Can you work these out from the model? Positions are in its coordinate system, mm. A direction names the side the tool comes from. Coordinates: 2 decimals unless noted, no trailing zeros. Order: outer loops, then holes, each group sorted by start corner. A loop starts at its lowest first (then second) coordinate and runs counter-clockwise, first axis right, second up. Notation, with made-up numbers: M 9.5,66.25 L 19.5,66.25 A22 cw 19.5,93.25 Z; hole C 53,15.25 d11. An arc over 180 degrees is marked long. Answer as a JSON object with one key per item and string values.
from build123d import *

# Parameters (mm, degrees)
SKETCH_1_W          = 29.8
SKETCH_1_H          = 29.8
SKETCH_1_W_2        = 25
SKETCH_1_H_2        = 25
EXTRUDE_1_DEPTH     = 40
SKETCH_2_R          = 8
SKETCH_2_R_2        = 5
EXTRUDE_1_2_DEPTH   = 10
SKETCH_3_R          = 8
EXTRUDE_2_DEPTH     = 4
FILLET_1_R          = 10
CUT_EXTRUDE_1_REACH = 58.671
SKETCH_4_R          = 2.2
SKETCH_5_R          = 5
CUT_EXTRUDE_2_DEPTH = 10
CUT_EXTRUDE_3_REACH = 52.454
SKETCH_6_W          = 25
SKETCH_6_H          = 25
SKETCH_7_R          = 3.2
SKETCH_7_R_2        = 1.2
EXTRUDE_3_DEPTH     = 4
FILLET_2_R          = 10


with BuildPart() as part:
    # Эскиз1 → Extrude 1 (new body)
    with BuildSketch(Plane(origin=(0, 0, 0), x_dir=(0, 0, -1), z_dir=(1, 0, 0))):
        Rectangle(SKETCH_1_W, SKETCH_1_H)
        Rectangle(SKETCH_1_W_2, SKETCH_1_H_2, mode=Mode.SUBTRACT)
    extrude(amount=EXTRUDE_1_DEPTH)

    # Эскиз2 → Extrude 1 2 (add)
    with BuildSketch(Plane(origin=(0, 14.9, 0), x_dir=(1, 0, 0), z_dir=(0, 1, 0))):
        with Locations((20, -18.9)):
            Circle(SKETCH_2_R)
        with Locations((20, -18.9)):
            Circle(SKETCH_2_R_2, mode=Mode.SUBTRACT)
    extrude(amount=-EXTRUDE_1_2_DEPTH)

    # Эскиз3 → Бобышка-Вытянуть2 (add)
    with BuildSketch(Plane.XZ.offset(-4.9)):
        with Locations((20, 18.9)):
            Circle(SKETCH_3_R)
    extrude(amount=EXTRUDE_2_DEPTH)

    # Скругление1
    fillet_1_edges = [part.edges().sort_by_distance(p)[0] for p in [
        (13.07179677, 7.9, 14.9),
        (26.92820323, 7.9, 14.9),
        (20, 0.9, 14.9),
    ]]
    fillet(fillet_1_edges, radius=FILLET_1_R)

    # Эскиз4 → Вырез-Вытянуть1 (cut, up to next)
    with BuildSketch(Plane(origin=(0, 14.9, 0), x_dir=(1, 0, 0), z_dir=(0, 1, 0)), mode=Mode.PRIVATE) as cut_extrude_1_sk1:
        with Locations(Location((10, 0, 0), (0, 0, 270))):
            Circle(SKETCH_4_R)
    cut_extrude_1_tool1 = extrude(cut_extrude_1_sk1.sketch, amount=-CUT_EXTRUDE_1_REACH, mode=Mode.PRIVATE) & part.part
    # Эскиз4 → Вырез-Вытянуть1 (cut, up to next)
    with BuildSketch(Plane(origin=(0, 14.9, 0), x_dir=(1, 0, 0), z_dir=(0, 1, 0)), mode=Mode.PRIVATE) as cut_extrude_1_sk2:
        with Locations(Location((30, 0, 0), (0, 0, 270))):
            Circle(SKETCH_4_R)
    cut_extrude_1_tool2 = extrude(cut_extrude_1_sk2.sketch, amount=-CUT_EXTRUDE_1_REACH, mode=Mode.PRIVATE) & part.part
    add(cut_extrude_1_tool1.solids().sort_by_distance((10, 14.9, 0))[0], mode=Mode.SUBTRACT)
    add(cut_extrude_1_tool2.solids().sort_by_distance((30, 14.9, 0))[0], mode=Mode.SUBTRACT)

    # Эскиз5 → Вырез-Вытянуть2 (cut)
    with BuildSketch(Plane(origin=(0, 14.9, 0), x_dir=(1, 0, 0), z_dir=(0, 1, 0))):
        with Locations(Location((20, -18.9, 0), (0, 0, 270))):
            Circle(SKETCH_5_R)
    extrude(amount=-CUT_EXTRUDE_2_DEPTH, mode=Mode.SUBTRACT)

    # Эскиз6 → Вырез-Вытянуть3 (cut, up to next)
    with BuildSketch(Plane(origin=(40, 0, 0), x_dir=(0, 0, -1), z_dir=(1, 0, 0)), mode=Mode.PRIVATE) as cut_extrude_3_sk1:
        Rectangle(SKETCH_6_W, SKETCH_6_H)
    cut_extrude_3_tool1 = extrude(cut_extrude_3_sk1.sketch, amount=-CUT_EXTRUDE_3_REACH, mode=Mode.PRIVATE) & part.part
    add(cut_extrude_3_tool1.solids().sort_by_distance((40, 0, 0))[0], mode=Mode.SUBTRACT)

    # Эскиз7 → Бобышка-Вытянуть3 (add)
    with BuildSketch(Plane.XZ.offset(14.9)):
        with Locations((20, -17.9)):
            Circle(SKETCH_7_R)
        with Locations(Location((20, -17.9, 0), (0, 0, 270))):
            Circle(SKETCH_7_R_2, mode=Mode.SUBTRACT)
    extrude(amount=-EXTRUDE_3_DEPTH)

    # Скругление2
    fillet_2_edges = [part.edges().sort_by_distance(p)[0] for p in [
        (18.886447127, -12.9, -14.9),
        (21.113552873, -12.9, -14.9),
    ]]
    fillet(fillet_2_edges, radius=FILLET_2_R)


solid = part.part
Item 1: I want a section at D-D, the plane z = 0. Write out the boundary of the cut face in (x, y).
Answers follow:
{"outline": "M 0,-14.9 L 40,-14.9 L 40,-12.5 L 0,-12.5 Z; M 0,12.5 L 7.8,12.5 L 7.8,14.9 L 0,14.9 Z; M 12.2,12.5 L 27.8,12.5 L 27.8,14.9 L 12.2,14.9 Z; M 32.2,12.5 L 40,12.5 L 40,14.9 L 32.2,14.9 Z"}
Item 2: I want a section at C-C, the plane z = -10. Write out the boundary of the cut face in (x, y), plus the area to 3 significant figures.
Answers follow:
{"outline": "M 0,-14.9 L 40,-14.9 L 40,-12.5 L 0,-12.5 Z; M 0,12.5 L 40,12.5 L 40,14.9 L 0,14.9 Z", "area": "192 mm^2"}
Item 3: I'm going to push flat-ended pins straight in: pin 1 (9 mm diameter, centred on x = 11, y = 1, fed in from +Z); pin 2 (8 mm diameter, centred on y = 4.5, z = -15.5, fed in from -X); pin 3 (4 mm diameter, centred on x = 10, z = 0, fed in from +Y); pin 4 (5 mm diameter, centred on x = 19.5, z = -19.5, fed in from +Y). Where does each tip first touch, or does it pass through?
Answers follow:
{"pin 1": "stops at z = 25.51", "pin 2": "stops at x = 0", "pin 3": "stops at y = -12.5", "pin 4": "stops at y = -10.9"}
Item 4: Please list where these lines run through material, in increasing order: line 1 (Y direction, x = 32, z = -6.5); line 2 (Z direction, x = 36.5, y = 1.5); line 3 (X direction, y = -13.15, z = -17.9).
Answers follow:
{"line 1": "y = -14.9 to -12.5, 12.5 to 14.9", "line 2": "z = -14.9 to -12.5, 12.5 to 14.91", "line 3": "x = 15.95 to 18.8, 21.2 to 24.05"}
Item 5: Which directions (+Z, -Z, +X, -X, +Y, -Y) give clear straight access to the entire face, cutting with the end or side of a thin tool? Please do faces 4 (the flat face through (20, -10, 14.9)), 5 (the cylindrical face through (21.66, 9.97, 14.184)), 6 (the flat face through (20, -10.9, -16)), 7 (the flat face through (20, 0, 12.5)).
Answers follow:
{"face 4": "+Z, -Y", "face 5": "+Y", "face 6": "-Z, +X, -X, +Y", "face 7": "+X, -X"}
Item 6: If we mould it in two halves opening along Y, with no side actions, what happens to faces 1 (the cylindrical face through (27.852, 13.717, -0.477)), 2 (the flat face through (20, 12.5, 0)), 3 (the flat face through (20, 0.9, 26))? For each: pulls with the +Y half, pulls with the -Y half, needs draft (parallel to the pull), parting line crosses it, or undercut.
Answers follow:
{"face 1": "needs draft", "face 2": "undercut", "face 3": "pulls with the -Y half"}
Item 7: I want a section at B-B, the plane x = 20. Write out the boundary of the cut face in (y, z).
Answers follow:
{"outline": "M -14.9,-21.1 L -10.9,-21.1 L -10.9,-19.1 L -14.9,-19.1 Z; M -14.9,-16.7 L -10.9,-16.7 L -10.9,-14.9 L 14.9,-14.9 L 14.9,13.9 L 4.9,13.9 L 4.9,23.9 L 14.9,23.9 L 14.9,26.9 L 0.9,26.9 L 0.9,24.9 A10 cw -9.1,14.9 L -14.9,14.9 Z; hole M -12.5,-12.5 L 12.5,-12.5 L 12.5,12.5 L -12.5,12.5 Z"}
Item 8: I want a section at A-A, the plane y = 8. Write out the boundary of the cut face in (x, z).
Answers follow:
{"outline": "M 0,-14.9 L 40,-14.9 L 40,-12.5 L 0,-12.5 Z; M 0,12.5 L 40,12.5 L 40,14.9 L 36.97,14.9 A10 cw 27.54,21.57 A8 ccw 12.46,21.57 A10 cw 3.03,14.9 L 0,14.9 Z; hole C 20,18.9 d10"}
